Part model, mm, in its own coordinate system. A direction names the side the tool comes from. Give positions to 0.01 mm unless a question says otherwise; leave off trailing zeros. Write each loop counter-clockwise with the first axis right and the second up, starting at its lowest first coordinate (ties: lowest second). Pieces come first, ordered by that corner, then holes.
Autodesk Inventor part; units mm, degrees
ref_plane "YZ Plane" through (0, 0, 0) normal (1, 0, 0) x (0, 1, 0)
ref_plane "XY Plane" through (0, 0, 0) normal (0, 0, 1) x (1, 0, 0)
ref_plane "UCS1: YZ Plane" through (0, 0, 0) normal (1, 0, 0) x (0, 1, 0)
sketch "Sketch2" plane through (0, 0, 0) normal (1, 0, 0) x (0, 1, 0)
  circle A0 centre (0, -70) radius 27.5
  line L0 (27.5, -190) -> (-27.5, -190)
  line L1 (0, -70) -> (0, -190) construction
  line L2 (-27.5, -70) -> (-27.5, -190)
  line L3 (27.5, -70) -> (27.5, -190)
  circle A1 centre (0, 0) radius 31
  line L4 (-30.9612, -1.55) -> (-27.4656, -71.375)
  line L5 (30.9612, -1.55) -> (27.4656, -71.375)
  line L6 (31.0388, 0) -> (-31.0388, 0)
  point P0 (-31, 0)
  point P1 (31, 0)
  point P2 (-31, 0)
  point P3 (-27.5, -70.6879)
  point P4 (27.5, -70.6879)
  dimension "d1" = 55
  dimension "d3" = 55
  dimension "d25" = 120
  dimension "d26" = 62
  dimension "d33" = 70
extrude "Extrusion1" add sketch "Sketch2" along normal blind 17.5 and the other way blind 32.5 contours A0
extrude "Extrusion2" add sketch "Sketch2" against normal blind 50 from surface at 17.5 contours L3 L5 A0 | A0 L4 L2 | L5 L3 L0 L2 L4 A0
sketch "Sketch5" plane through (17.5, -27.5, -190) normal (0, 0, -1) x (-1, 0, 0)
  circle A0 centre (25, 27.5) radius 10
  line L0 (50, 55) -> (50, 0)
  line L1 (0, 55) -> (50, 55)
  point P0 (17.5, 27.5)
  point P1 (50, 27.5)
  point P2 (-45, 0)
  point P3 (25, 55)
  dimension "d22" = 20
extrude "Extrusion4" cut sketch "Sketch5" against normal blind 60
ref_plane "Work Plane1" through (-7.5, 0, -70) normal (-1, 0, 0) x (0, 0, -1)
sketch "Sketch4" plane through (-7.5, 0, -70) normal (-1, 0, 0) x (0, 0, -1)
  circle A0 centre (-70, 0) radius 190
  line L0 (120, -27.5) -> (120, 27.5)
  line L1 (-260, 0) -> (120, 0)
  line L2 (120, 0) -> (120, 27.5)
  line L3 (120, 27.5) -> (0, 27.5)
  line L4 (120, 27.5) -> (120, 47.2424)
  line L5 (120, 47.2424) -> (114.033, 47.2424)
  point P0 (-70, 0)
  point P1 (117.9993, 27.5)
  point P2 (120, 0)
revolve "Revolution1" cut sketch "Sketch4" angle 360 about axis through (-7.5, 0, 190) along (0, 0, -1) contours L5 L4 L3 A0 | L3 L0 A0
extrude "Extrusion5" add sketch "Sketch2" along normal blind 17.5 and the other way blind 32.5 contours A0 L2 L4 A1 L5 L3
properties part number "shank_inventor"
1) Saw through at A-A (z = -172). Write the cut outline in (x, y).
Check result:
outline: (-32.5, -27.5) - (17.5, -27.5) - (17.5, 27.5) - (-32.5, 27.5) - close; hole circle Ø20 at (-7.5, 0)
2) 3-axis set-ups, long thin cutter, end or side, ignore diameter. For faces 1 (the cylindrical face through (-7.85, 0.66, -30.993)), 2 (the flat face through (-7, 27.5, -129)): which of +Z, -Z, +X, -X, +Y, -Y reach the whole face in a straight line?
Check result:
face 1: +Z, +X, -X
face 2: -Z, +X, -X, +Y
3) Saw through at D-D (x = -7.5). Write the cut outline in (y, z), and give its area (3 significant figures).
Check result:
outline: (-30.96, -1.59) - (-27.5, -70.69) - (-27.5, -188) arc R190 ccw to (-10, -189.74) - (-10, -130) - (10, -130) - (10, -189.74) arc R190 ccw to (27.5, -188) - (27.5, -70.69) - (30.96, -1.59) arc R31 cw to start
area: 7,960 mm2
4) Mould opens along X. For faces 3 (the flat face through (17.5, 0, -94)), 4 (the flat face through (-7, 0, -130)), 5 (the flat face through (-7, -27.5, -129)), 6 (the cylindrical face through (2.49, 0.44, -160.29)) say: +X half, -X half, draft (parallel to the pull), parting line (faces both ways), or undercut.
Check result:
face 3: +X half
face 4: undercut
face 5: draft
face 6: undercut
5) Saw through at C-C (z = -21.5). Write the cut outline in (x, y).
Check result:
outline: (-32.5, -29.96) - (17.5, -29.96) - (17.5, -22.33) - (-32.5, -22.33) - close; (-32.5, 22.33) - (17.5, 22.33) - (17.5, 29.96) - (-32.5, 29.96) - close
6) Drill centre lines: L1, parallel to X at y = 0, z = -141.5; L2, parallel to Y at x = -7.5, z = -158; L3, parallel to Y at x = -28, z = -135. Where is each one in solid material? Low to high.
Check result:
L1: x = -32.5 to -17.5, 2.5 to 17.5
L2: y = -27.5 to -10, 10 to 27.5
L3: y = -27.5 to 27.5
7) Saw through at B-B (y = 0). Write the cut outline in (x, z), and give its area (3 significant figures).
Check result:
outline: (-32.5, -188.35) arc R190 ccw to (-17.5, -189.74) - (-17.5, -130) - (2.5, -130) - (2.5, -189.74) arc R190 ccw to (17.5, -188.35) - (17.5, -31) - (-32.5, -31) - close
area: 6,720 mm2
8) Flat gauge pins, fed straight in: P1, Ø5, axis at x = -1.5, z = -62, coming from the +Y side; P2, Ø1, axis at x = -20, y = 24, coming from the -Z side; P3, Ø12, axis at x = -7.5, y = 0, coming from the -Z side. Where does each tip first touch, or does it go through?
Check result:
P1: stops at y = 28.06
P2: stops at z = -188.13
P3: stops at z = -130
